Can you work these out from the model? Positions are in its coordinate system, mm. A direction names the side the tool comes from. Round coordinates to 2 decimals unless told otherwise and drop trailing zeros. Order: outer loops, then holes, each group sorted by start corner. A loop starts at its lowest first (then second) coordinate and runs counter-clockwise, first axis right, second up. Notation, with made-up numbers: (71, 43) -> (110, 43) arc R15 ccw to (110, 64) -> close; hole circle Ø2 at (11, 42.25). An arc over 180 degrees is marked (long way). One line per item, written item: value.
```python
from build123d import *

# Parameters (mm, degrees)
F0_W     = 17
F0_H     = 17
F1_DEPTH = 10
F3_DEPTH = 2


with BuildPart() as f1:
    # F0 (on Front) → F1 (new body, symmetric)
    with BuildSketch(Plane.XZ):
        Polygon((-20, 41), (-20, 0), (21, 0), (21, 60), (-1, 60), (-1, 41), align=None)
        with Locations((-9.5, 11.5)):
            Rectangle(F0_W, F0_H, mode=Mode.SUBTRACT)
        with Locations((9.5, 11.5)):
            Rectangle(F0_W, F0_H, mode=Mode.SUBTRACT)
        with Locations((-9.5, 30.5)):
            Rectangle(F0_W, F0_H, mode=Mode.SUBTRACT)
        with Locations((9.5, 30.5)):
            Rectangle(F0_W, F0_H, mode=Mode.SUBTRACT)
        with Locations((9.5, 49.5)):
            Rectangle(F0_W, F0_H, mode=Mode.SUBTRACT)
    extrude(amount=F1_DEPTH, both=True)

    # F2 (on Front) → F3 (join, symmetric)
    with BuildSketch(Plane.XZ):
        Polygon((-1, 57.87868), (-1, 60), (-20, 41), (-17.87868, 41), align=None)
    extrude(amount=F3_DEPTH, both=True)


solid = f1.part
```
Q1. Will these pins go through, and if not, where does the flat tip stop? pin 1 Ø4 at (x, z) = (-15.5, 44) entering from +Y; pin 2 Ø5 at (x, y) = (-4.5, 0) entering from +Z; pin 3 Ø8.5 at (x, y) = (-10, 1.5) entering from +Z.
Answers below:
pin 1: y = 2
pin 2: z = 59
pin 3: z = 55.25
Q2. We'd pull the mould along X, two halves only. Please class faces 3 (the face through (21, 0, 30)), 4 (the face through (-10, 0, 51)), 5 (the face through (9, 0, 22)), 6 (the face through (-1, 0, 11)): released by +X, released by -X, zero draft, split by the parting line, or undercut.
Answers below:
face 3: released by +X
face 4: released by -X
face 5: undercut
face 6: undercut
Q3. I want a section at D-D on z = 43. List the corners of the cut face in (x, y) for me, plus the area to 3 significant figures.
Answers below:
outline: (-18, -2) -> (-15.88, -2) -> (-15.88, 2) -> (-18, 2) -> close; (-1, -10) -> (1, -10) -> (1, 10) -> (-1, 10) -> close; (18, -10) -> (21, -10) -> (21, 10) -> (18, 10) -> close
area: 108 mm^2
Q4. I want a section at A-A on z = 7. List the corners of the cut face in (x, y) for me, plus the area to 3 significant figures.
Answers below:
outline: (-20, -10) -> (-18, -10) -> (-18, 10) -> (-20, 10) -> close; (-1, -10) -> (1, -10) -> (1, 10) -> (-1, 10) -> close; (18, -10) -> (21, -10) -> (21, 10) -> (18, 10) -> close
area: 140 mm^2
Q5. I want a section at C-C on y = 5. List the corners of the cut face in (x, z) for me, plus the area to 3 significant figures.
Answers below:
outline: (-20, 0) -> (21, 0) -> (21, 60) -> (-1, 60) -> (-1, 41) -> (-20, 41) -> close; hole (-18, 3) -> (-1, 3) -> (-1, 20) -> (-18, 20) -> close; hole (-18, 22) -> (-1, 22) -> (-1, 39) -> (-18, 39) -> close; hole (1, 3) -> (18, 3) -> (18, 20) -> (1, 20) -> close; hole (1, 22) -> (18, 22) -> (18, 39) -> (1, 39) -> close; hole (1, 41) -> (18, 41) -> (18, 58) -> (1, 58) -> close
area: 654 mm^2
Q6. I want a section at B-B on x = 16. List the corners of the cut face in (y, z) for me.
Answers below:
outline: (-10, 0) -> (10, 0) -> (10, 3) -> (-10, 3) -> close; (-10, 20) -> (10, 20) -> (10, 22) -> (-10, 22) -> close; (-10, 39) -> (10, 39) -> (10, 41) -> (-10, 41) -> close; (-10, 58) -> (10, 58) -> (10, 60) -> (-10, 60) -> close
Q7. Please list where these lines run through material, in increasing order: line 1 along Z through (x, y) = (3.5, -8.75); line 2 along Z through (x, y) = (-6.5, -8.25); line 3 along X through (y, z) = (1.5, 8).
Answers below:
line 1: 0 to 3, 20 to 22, 39 to 41, 58 to 60
line 2: 0 to 3, 20 to 22, 39 to 41
line 3: -20 to -18, -1 to 1, 18 to 21
Q8. On a 3-axis mill with a long thin cutter (end or side, diameter ignored), from which of +Z, -Z, +X, -X, +Y, -Y can I reach the whole of each face in a straight line? I mean faces 1 (the face through (0, 0, 0)), 2 (the face through (9, 0, 39)). Say none if no direction works.
Answers below:
face 1: -Z, +X, -X, +Y, -Y
face 2: +Y, -Y
